Check sheet for the modelled part. Datum: model origin and axes. Units: mm. A direction names the side the tool comes from. Coordinates: 2 decimals unless noted, no trailing zeros. Loops run counter-clockwise (first coordinate to the right, second up) from the corner with the lowest first, then second, coordinate; pieces in that order, holes last. Notation, with made-up numbers: (-6, 4) -> (9, 4) arc R22 cw to (9, 41) -> close; hole circle Ø11 at (54, 75). An arc over 180 degrees is marked (long way). Use CSV: the item, a comma, the result in double quotes. Start each with the question number.
1. Sectioned sample at A-A, the plane y = 9. Record the cut outline in (x, z), and give its area (3 significant figures).
2. Gauge pin test, flat ends, axial feed: pin 1 (3 mm diameter, centred on y = 5.5, z = 22, fed in from +X); pin 2 (1 mm diameter, centred on x = -67.5, y = 16.5, fed in from -Z); pin 3 (8 mm diameter, centred on x = -16.5, y = 25.5, fed in from +Z). Record the tip position at first contact, or that the pin passes through.
3. Sectioned sample at B-B, the plane x = -50. Record the cut outline in (y, z).
4. Set-up check for faces 1 (the face through (-50, 20, 3)), 2 (the face through (-70, 5, 23)), 3 (the face through (-30, 5, 22)), 4 (the face through (-50, 10, 28)): record each of +Z, -Z, +X, -X, +Y, -Y from which the full face is reachable in a straight line by a thin tool's end or side.
5. Sectioned sample at D-D, the plane z = 47. Record the cut outline in (x, y).
6. Thickness scan on L1, parallel to Z at x = -50, y = 3.5; L2, parallel to Y at x = -69.5, z = 23. Record the ranges inside material, lowest first.
7. Sectioned sample at C-C, the plane y = 26. Record the cut outline in (x, z).
```python
from build123d import *

# Parameters (mm, degrees)
F0_W     = 100
F0_H     = 40
F1_DEPTH = 10
F2_W     = 40
F2_H     = 10
F3_DEPTH = 10
F4_W     = 40
F4_H     = 3
F5_DEPTH = 40.001
F6_R     = 2.25
F7_DEPTH = 40.001


with BuildPart() as f1:
    # F0 (on Top) → F1 (new body)
    with BuildSketch(Plane.XY):
        with Locations((-50, 20)):
            Rectangle(F0_W, F0_H)
    extrude(amount=F1_DEPTH)

    # F2 (on face) → F3 (join)
    with BuildSketch(Plane.XZ):
        with BuildLine():
            Line((-70, 35), (-70, 10))
            Line((-70, 10), (-30, 10))
            Line((-30, 10), (-30, 35))
            ThreePointArc((-30, 35), (-50, 55), (-70, 35))
        make_face()
        with Locations((-50, 5)):
            Rectangle(F2_W, F2_H)
    extrude(amount=-F3_DEPTH)

    # F4 (on face) → F5 (cut, through all)
    with BuildSketch(Plane.XZ):
        with Locations((-50, 1.5)):
            Rectangle(F4_W, F4_H)
    extrude(amount=-F5_DEPTH, mode=Mode.SUBTRACT)

    # F6 (on face) → F7 (cut, through all)
    with BuildSketch(Plane.XZ):
        with Locations((-50, 35)):
            Circle(F6_R)
    extrude(amount=-F7_DEPTH, mode=Mode.SUBTRACT)


solid = f1.part
```
Completed:
1,outline,"(-100, 0) -> (-70, 0) -> (-70, 3) -> (-30, 3) -> (-30, 0) -> (0, 0) -> (0, 10) -> (-30, 10) -> (-30, 35) arc R20 ccw to (-70, 35) -> (-70, 10) -> (-100, 10) -> close; hole circle Ø4.5 at (-50, 35)"
1,area,"2,490 mm²"
2,pin 1,"x = -30"
2,pin 2,"z = 3"
2,pin 3,"z = 10"
3,outline,"(0, 3) -> (40, 3) -> (40, 10) -> (10, 10) -> (10, 32.75) -> (0, 32.75) -> close; (0, 37.25) -> (10, 37.25) -> (10, 55) -> (0, 55) -> close"
4,face 1,"-Z, +Y, -Y"
4,face 2,"+Z, -X, +Y, -Y"
4,face 3,"+Z, +X, +Y, -Y"
4,face 4,"+Z, +X, -X, +Y"
5,outline,"(-66, 0) -> (-34, 0) -> (-34, 10) -> (-66, 10) -> close"
6,L1,"3 to 32.75, 37.25 to 55"
6,L2,"0 to 10"
7,outline,"(-100, 0) -> (-70, 0) -> (-70, 3) -> (-30, 3) -> (-30, 0) -> (0, 0) -> (0, 10) -> (-100, 10) -> close"
